Geometry check sheet. Reference: the model listing, model coordinates, mm. Face numbers are marked on the shaded views. A direction names the side the tool comes from. Round coordinates to 2 decimals unless told otherwise and drop trailing zeros. Write each loop counter-clockwise with the first axis right and the second up, starting at its lowest first coordinate (ties: lowest second). Pieces come first, ordered by that corner, then holes. Notation, with made-up numbers: (18, 19) - (48, 19) arc R28 cw to (48, 38) - close; hole circle Ø2 at (54, 24). An arc over 180 degrees is marked (long way). Return JSON: item names as keys, results as strings.
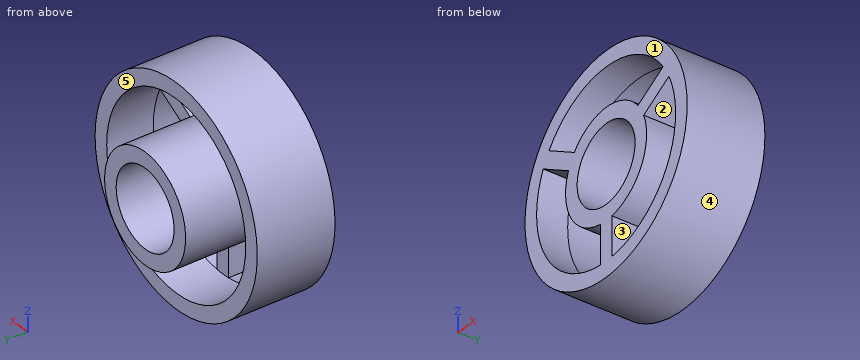
```python
from build123d import *

# Parameters (mm, degrees)
SKETCH1_R           = 7
BOSS_EXTRUDE1_DEPTH = 5
SKETCH2_R           = 6
CUT_EXTRUDE1_DEPTH  = 3
SKETCH3_R           = 3.5
BOSS_EXTRUDE3_DEPTH = 5
SKETCH4_R           = 2.5
CUT_EXTRUDE2_DEPTH  = 8
CUT_EXTRUDE3_DEPTH  = 3


with BuildPart() as part:
    # Sketch1 → Boss-Extrude1 (new body)
    with BuildSketch(Plane(origin=(0, 0, 0), x_dir=(1, 0, 0), z_dir=(0, 1, 0))):
        Circle(SKETCH1_R)
    extrude(amount=BOSS_EXTRUDE1_DEPTH)

    # Sketch2 → Cut-Extrude1 (cut)
    with BuildSketch(Plane(origin=(0, 5, 0), x_dir=(1, 0, 0), z_dir=(0, 1, 0))):
        Circle(SKETCH2_R)
    extrude(amount=-CUT_EXTRUDE1_DEPTH, mode=Mode.SUBTRACT)

    # Sketch3 → Boss-Extrude3 (add)
    with BuildSketch(Plane(origin=(0, 2, 0), x_dir=(1, 0, 0), z_dir=(0, 1, 0))):
        Circle(SKETCH3_R)
    extrude(amount=BOSS_EXTRUDE3_DEPTH)

    # Sketch4 → Cut-Extrude2 (cut, through all)
    with BuildSketch(Plane(origin=(0, 7, 0), x_dir=(1, 0, 0), z_dir=(0, 1, 0))):
        Circle(SKETCH4_R)
    extrude(amount=-CUT_EXTRUDE2_DEPTH, mode=Mode.SUBTRACT)

    # Sketch5 → Cut-Extrude3 (cut, through all)
    with BuildSketch(Plane(origin=(0, 2, 0), x_dir=(1, 0, 0), z_dir=(0, 1, 0))):
        with BuildLine():
            Line((-0.5, 5.979130372), (-0.5, 3.464101615))
            ThreePointArc((-0.5, 3.464101615), (-3.031088913, 1.75), (-3.25, -1.299038106))
            Line((-3.25, -1.299038106), (-5.428078794, -2.556552484))
            ThreePointArc((-5.428078794, -2.556552484), (-5.196152423, 3), (-0.5, 5.979130372))
        make_face()
        with BuildLine():
            Line((0.5, 5.979130372), (0.5, 3.464101615))
            ThreePointArc((0.5, 3.464101615), (3.031088913, 1.75), (3.25, -1.299038106))
            Line((3.25, -1.299038106), (5.428078794, -2.556552484))
            ThreePointArc((5.428078794, -2.556552484), (5.196152423, 3), (0.5, 5.979130372))
        make_face()
        with BuildLine():
            Line((-4.928078794, -3.422577888), (-2.75, -2.165063509))
            ThreePointArc((-2.75, -2.165063509), (0, -3.5), (2.75, -2.165063509))
            Line((2.75, -2.165063509), (4.928078794, -3.422577888))
            ThreePointArc((4.928078794, -3.422577888), (0, -6), (-4.928078794, -3.422577888))
        make_face()
    extrude(amount=-CUT_EXTRUDE3_DEPTH, mode=Mode.SUBTRACT)


solid = part.part
```
(1) Section check C-C, the plane y = 4.5. Enter the section's corners in (x, z).
Response values:
{"outline": "circle Ø14 at (0, 0); circle Ø7 at (0, 0); hole circle Ø12 at (0, 0); hole circle Ø5 at (0, 0)"}
(2) Section check A-A, the plane z = 0. Enter the section's corners in (x, y), plus the area to 3 significant figures.
Response values:
{"outline": "(-7, 0) - (-6, 0) - (-6, 5) - (-7, 5) - close; (-3.5, 0) - (-2.5, 0) - (-2.5, 7) - (-3.5, 7) - close; (2.5, 0) - (3.5, 0) - (3.5, 7) - (2.5, 7) - close; (6, 0) - (7, 0) - (7, 5) - (6, 5) - close", "area": "24.0 mm^2"}
(3) Material ranges on line 1 along X through (y, z) = (3.25, 0); line 2 along X through (y, z) = (3, 2.25), recorded low to high. Write a range as [from, to].
Response values:
{"line 1": "x = [-7, -6], [-3.5, -2.5], [2.5, 3.5], [6, 7]", "line 2": "x = [-6.63, -5.56], [-2.68, -1.09], [1.09, 2.68], [5.56, 6.63]"}
(4) Section check B-B, the plane x = 0. Enter the section's corners in (y, z), plus the area to 3 significant figures.
Response values:
{"outline": "(0, -7) - (5, -7) - (5, -6) - (2, -6) - (2, -3.5) - (7, -3.5) - (7, -2.5) - (0, -2.5) - close; (0, 2.5) - (7, 2.5) - (7, 3.5) - (0, 3.5) - close; (0, 6) - (5, 6) - (5, 7) - (0, 7) - close", "area": "29.0 mm^2"}
(5) Gauge pin test, flat ends, axial feed: pin 1 (1.7 mm diameter, centred on x = -4, z = 2.5, fed in from +Y); pin 2 (0.6 mm diameter, centred on y = 1, z = -4.5, fed in from +X); pin 3 (2 mm diameter, centred on x = -1.5, z = -2, fed in from -Y); pin 4 (2 mm diameter, centred on x = -2.5, y = 1, fed in from +Z). Record the tip position at first contact, or that the pin passes through.
Response values:
{"pin 1": "stops at y = 2", "pin 2": "stops at x = 5.6", "pin 3": "stops at y = 0", "pin 4": "stops at z = 6.84"}
(6) Access from +Z, -Z, +X, -X, +Y, -Y to the whole of each face (thin tool, end or side, straight path). Record for the marked faces 1 and 2.
Response values:
{"face 1": "+Z, -Z, +X, -X, -Y", "face 2": "+Y, -Y"}
(7) Release check for a two-part mould opening along X. For the marked faces 3, 4 and 5 record: pulls with the +X half, pulls with the -X half, needs draft (parallel to the pull), parting line crosses it, or undercut.
Response values:
{"face 3": "undercut", "face 4": "parting line crosses it", "face 5": "needs draft"}
(8) Section check D-D, the plane z = 4.75. Enter the section's corners in (x, y), plus the area to 3 significant figures.
Response values:
{"outline": "(-5.14, 0) - (-3.67, 0) - (-3.67, 5) - (-5.14, 5) - close; (3.67, 0) - (5.14, 0) - (5.14, 5) - (3.67, 5) - close", "area": "14.8 mm^2"}
